```python
from build123d import *

# Parameters (mm, degrees)
SKIZZE1_W                       = 15
SKIZZE1_H                       = 10
SKIZZE1_R                       = 1.6
AUFSATZ_LINEAR_AUSTRAGEN1_DEPTH = 5
SKIZZE1_9_W                     = 5
SKIZZE1_9_H                     = 10
AUFSATZ_LINEAR_AUSTRAGEN2_DEPTH = 20
SKIZZE3_R                       = 1.6
SCHNITT_LINEAR_AUSTRAGEN2_DEPTH = 20
FASE2_SIZE                      = 3


with BuildPart() as part:
    # Skizze1 → Aufsatz-Linear austragen1 (new body)
    with BuildSketch(Plane.XY):
        with Locations((12.5, 5)):
            Rectangle(SKIZZE1_W, SKIZZE1_H)
        with Locations((15, 5)):
            Circle(SKIZZE1_R, mode=Mode.SUBTRACT)
    extrude(amount=AUFSATZ_LINEAR_AUSTRAGEN1_DEPTH)

    # Skizze1_9 → Aufsatz-Linear austragen2 (add)
    with BuildSketch(Plane.XY):
        with Locations((2.5, 5)):
            Rectangle(SKIZZE1_9_W, SKIZZE1_9_H)
    extrude(amount=AUFSATZ_LINEAR_AUSTRAGEN2_DEPTH)

    # Skizze3 → Schnitt-Linear austragen2 (cut)
    with BuildSketch(Plane(origin=(5, 0, 0), x_dir=(0, 0, -1), z_dir=(1, 0, 0))):
        with Locations(Location((-15, 5, 0), (0, 0, 90))):
            Circle(SKIZZE3_R)
    extrude(amount=-SCHNITT_LINEAR_AUSTRAGEN2_DEPTH, mode=Mode.SUBTRACT)

    # Fase2
    fase2_edges = [part.edges().sort_by_distance(p)[0] for p in [
        (5, 5, 20),
        (20, 5, 5),
        (5, 5, 5),
    ]]
    chamfer(fase2_edges, length=FASE2_SIZE)


solid = part.part
```
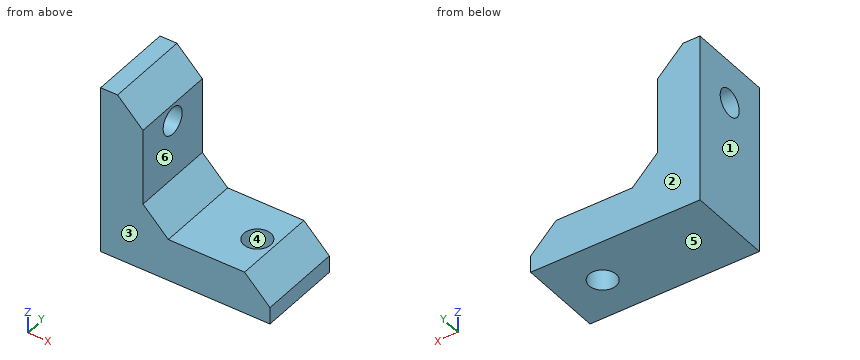
Build history of the part. All positions in model axes, mm. Face numbers are marked on the shaded views. A direction names the side the tool comes from. Give positions to 0.01 mm unless a question says otherwise; leave off trailing zeros. Order: outer loops, then holes, each group sorted by start corner. A loop starts at its lowest first (then second) coordinate and runs counter-clockwise, first axis right, second up. Notation, with made-up numbers: M 38,-2.5 L 73,-2.5 A18 cw 73,26.5 Z; hole C 78,-33 d2. An arc over 180 degrees is marked long. Return JSON: item names as keys, results as strings.
Q1. Two-plate mould, pull along Y, no slides. Class the marked faces 1, 2, 3 and 4: pulls with the +Y half, pulls with the -Y half, needs draft (parallel to the pull), parting line crosses it, or undercut.
Answer list:
{"face 1": "needs draft", "face 2": "pulls with the +Y half", "face 3": "pulls with the -Y half", "face 4": "undercut"}
Q2. Band-saw the part on B-B (z = 15). Give the cut face in (x, y), then the cut area to 3 significant figures.
Answer list:
{"outline": "M 0,0 L 5,0 L 5,3.4 L 0,3.4 Z; M 0,6.6 L 5,6.6 L 5,10 L 0,10 Z", "area": "34.0 mm^2"}
Q3. 3-axis set-ups, long thin cutter, end or side, ignore diameter. For the marked faces 5 and 6: which of +Z, -Z, +X, -X, +Y, -Y reach the whole face in a straight line?
Answer list:
{"face 5": "-Z, +X, -X, +Y, -Y", "face 6": "+Z, +X, +Y, -Y"}
Q4. Wall check: probe 1 along Y at (x, z) = (15, 3.05); probe 2 along X at (y, z) = (0.5, 12.75); probe 3 along Z at (x, y) = (3.85, 5). Give the ranges that are in metal, low to high. Write a range as from..to.
Answer list:
{"probe 1": "y = 0..3.4, 6.6..10", "probe 2": "x = 0..5", "probe 3": "z = 0..13.4, 16.6..18.15"}
Q5. Flat gauge pins, fed straight in: pin 1 (4 mm diameter, centred on x = 15, y = 5, fed in from +Z); pin 2 (3.5 mm diameter, centred on y = 5, z = 15, fed in from +X); pin 3 (12 mm diameter, centred on x = 14.5, z = 18, fed in from -Y); pin 4 (2 mm diameter, centred on y = 2.5, z = 8.5, fed in from +X). Where does each tip first touch, or does it go through?
Answer list:
{"pin 1": "stops at z = 5", "pin 2": "stops at x = 5", "pin 3": "passes through", "pin 4": "stops at x = 5.5"}
Q6. Band-saw the part on C-C (x = 15). Give the cut face in (y, z), then the cut area to 3 significant figures.
Answer list:
{"outline": "M 0,0 L 3.4,0 L 3.4,5 L 0,5 Z; M 6.6,0 L 10,0 L 10,5 L 6.6,5 Z", "area": "34.0 mm^2"}
Q7. Band-saw the part on A-A (y = 5). Give the cut face in (x, z), then the cut area to 4 significant figures.
Answer list:
{"outline": "M 0,0 L 13.4,0 L 13.4,5 L 8,5 L 5,8 L 5,13.4 L 0,13.4 Z; M 0,16.6 L 5,16.6 L 5,17 L 2,20 L 0,20 Z; M 16.6,0 L 20,0 L 20,2 L 17,5 L 16.6,5 Z", "area": "138.5 mm^2"}
Q8. Band-saw the part on D-D (y = 2). Give the cut face in (x, z), then the cut area to 4 significant figures.
Answer list:
{"outline": "M 0,0 L 20,0 L 20,2 L 17,5 L 8,5 L 5,8 L 5,17 L 2,20 L 0,20 Z", "area": "170.5 mm^2"}
